Geometry check sheet. Reference: the model listing, model coordinates, mm. Round coordinates to 2 decimals unless told otherwise and drop trailing zeros. Loops run counter-clockwise (first coordinate to the right, second up) from the corner with the lowest first, then second, coordinate; pieces in that order, holes last. Notation, with made-up numbers: (12.25, 83.25) - (69.25, 83.25) arc R26 cw to (69.25, 120.25) - close; hole circle Ø3 at (-32.75, 20). An arc over 180 degrees is marked (long way). Answer in a Markdown table with one row per item. Add a question column.
Autodesk Inventor part; units mm, degrees
ref_plane "YZ Plane" through (0, 0, 0) normal (1, 0, 0) x (0, 1, 0)
ref_plane "XZ Plane" through (0, 0, 0) normal (0, 1, 0) x (-1, 0, 0)
ref_plane "XY Plane" through (0, 0, 0) normal (0, 0, 1) x (1, 0, 0)
sketch "Sketch1" plane through (0, 0, 0) normal (0, 0, 1) x (1, 0, 0)
  circle A0 centre (-2.6438, 6.9447) radius 6.8758
  line L0 (-9.4616, 7.8359) -> (-6.8245, 12.4034)
  line L1 (-6.8245, 1.4859) -> (-9.4616, 6.0534)
  line L2 (-0.0068, 0.5947) -> (-5.2808, 0.5947)
  line L3 (4.174, 6.0534) -> (1.537, 1.4859)
  line L4 (1.537, 12.4034) -> (4.174, 7.8359)
  line L5 (-5.2808, 13.2947) -> (-0.0068, 13.2947)
  point P0 (0, 0)
  point P1 (1.537, 1.4859)
  dimension "d0" = 13.7516
  dimension "d4" = 360
extrude "Extrusion1" add sketch "Sketch1" along normal blind 273.05 contours A0 L3 L2 L1 L0 L5 L4
sketch "Sketch2" plane through (0, 0, 273.05) normal (0, 0, 1) x (1, 0, 0)
  circle A0 centre (-2.6438, 6.9447) radius 2.5527
  line L0 (-5.2808, 0.5947) -> (-0.0068, 0.5947)
  line L1 (-2.6438, 6.9447) -> (-5.2808, 0.5947) construction
  line L2 (-2.6438, 6.9447) -> (-0.0068, 0.5947) construction
  point P0 (0, 0)
  dimension "d8" = 5.1054
  dimension "d9" = 6.35
extrude "Extrusion2" cut sketch "Sketch2" against normal blind 273.05
equation "\"d6\" = d5"
equation "\"d10\" = d5"
equation "\"d5\" = 273.05"
properties part number "10.75in THUNDERSHAFT"
Q1. Cross-section at B-B, the plane z = 223.5. Enter the section's corners in (x, y), plus the area to 3 significant figures.
Q2. Scan lines: line 1 (X direction, y = 7, z = 227.5); line 2 (Y direction, x = -2.5, z = 214.5); line 3 (Y direction, x = 0, z = 133.5). Record each from-to range of solid material in increasing order. Write a range as from..to.
Q3. Cross-section at A-A, the plane x = -2.5. Enter the section's corners in (y, z), plus the area to 3 significant figures.
Q4. Release check for a two-part mould opening along X. For faces 1 (the flat face through (-3, 10, 273.05)), 2 (the flat face through (2.84, 10.15, 134.61)), 3 (the cylindrical face through (-1.271, 9.097, 138.436)), 4 (the flat face through (-8.125, 3.738, 134.614)) record: +X half, -X half, draft (parallel to the pull), parting line (faces both ways), or undercut.
Q5. Depth check by flat-ended pin: P1, Ø1.5, axis at y = 2.5, z = 177, coming from the -X side; P2, Ø1, axis at x = 2, z = 37.5, coming from the +Y side; P3, Ø3, axis at x = -2.64, y = 6.94, coming from the +Z side; P4, Ø8, axis at x = 0.5, z = 213, coming from the +Y side. Enter the tip coordinate at first touch or a pass-through.
Check sheet entries:
| question | item | result |
|---|---|---|
| 1 | outline | (-9.46, 6.05) - (-6.82, 1.49) arc R6.88 ccw to (-5.28, 0.59) - (-0.01, 0.59) arc R6.88 ccw to (1.54, 1.49) - (4.17, 6.05) arc R6.88 ccw to (4.17, 7.84) - (1.54, 12.4) arc R6.88 ccw to (-0.01, 13.29) - (-5.28, 13.29) arc R6.88 ccw to (-6.82, 12.4) - (-9.46, 7.84) arc R6.88 ccw to start; hole circle Ø5.11 at (-2.64, 6.94) |
| 1 | area | 117 mm² |
| 2 | line 1 | -9.52..-5.2, -0.09..4.23 |
| 2 | line 2 | 0.59..4.4, 9.49..13.29 |
| 2 | line 3 | 0.6..13.29 |
| 3 | outline | (0.59, 0) - (4.4, 0) - (4.4, 273.05) - (0.59, 273.05) - close; (9.49, 0) - (13.29, 0) - (13.29, 273.05) - (9.49, 273.05) - close |
| 3 | area | 2,080 mm² |
| 4 | face 1 | draft |
| 4 | face 2 | +X half |
| 4 | face 3 | undercut |
| 4 | face 4 | -X half |
| 5 | P1 | x = -7.84 |
| 5 | P2 | y = 12.43 |
| 5 | P3 | through |
| 5 | P4 | y = 13.29 |
